Geometry: see drawing. Coordinates: mm, zero at the bounding-box minimum. A direction names the side the tool comes from. Give positions to 0.01 mm unless a question says otherwise; leave off trailing zeros. Order: outer loops, then holes, each group sorted by start corner. A loop starts at its lowest first (then second) coordinate and runs counter-clockwise, first axis right, second up. Notation, with made-up numbers: M 36,-5.5 L 48,-5.5 A21 ccw 48,15.5 Z; hole C 85,36.25 d3. An arc over 180 degrees is marked long. Use a Markdown table: item, result.
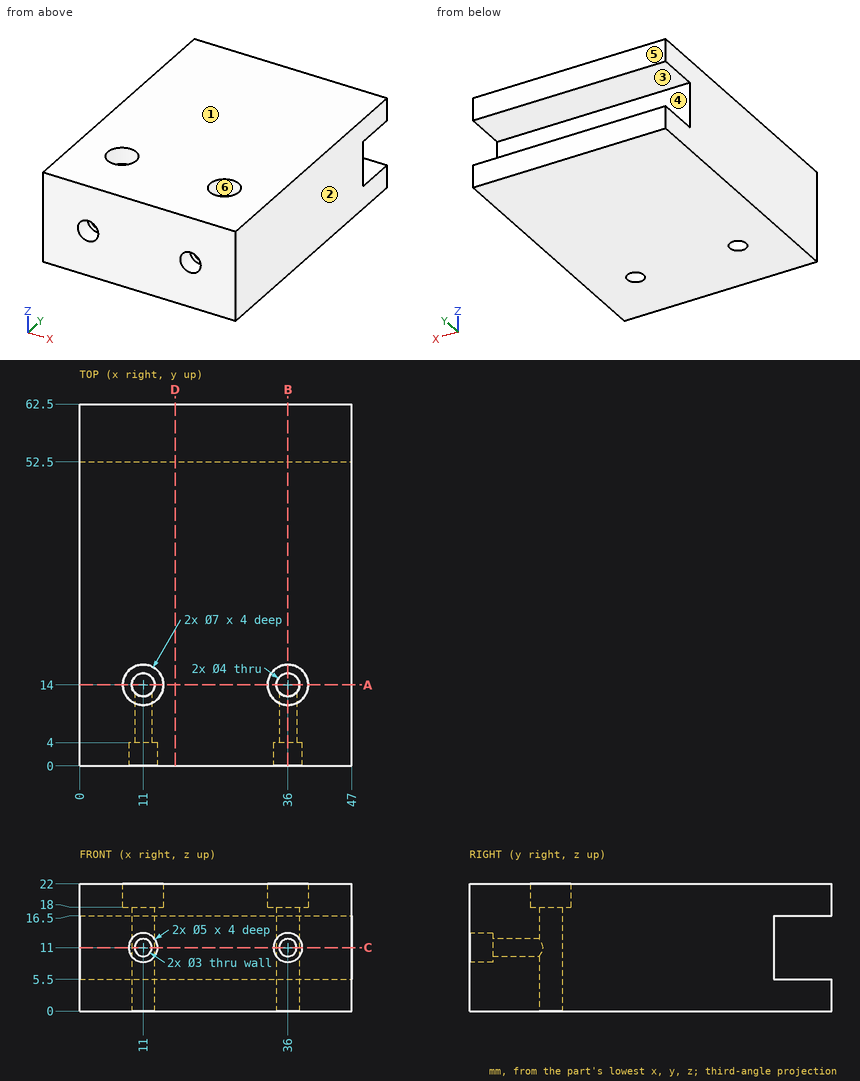
1) Cut plane D-D on x = 16.5. Return loops of the section in (y, z).
Response values:
| item | result |
|---|---|
| outline | M 0,0 L 62.5,0 L 62.5,5.5 L 52.5,5.5 L 52.5,16.5 L 62.5,16.5 L 62.5,22 L 0,22 Z |
2) Material intervals for line 1 (X direction, y = 14, z = 20.5); line 2 (X direction, y = 14, z = 11.5); line 3 (Z direction, x = 11, y = 7.5), sorted ascending. Write a range as from..to.
Response values:
| item | result |
|---|---|
| line 1 | x = 0..7.5, 14.5..32.5, 39.5..47 |
| line 2 | x = 0..9, 13..34, 38..47 |
| line 3 | z = 0..9.5, 12.5..22 |
3) Reachability of the marked faces 5 and 6 from +Z, -Z, +X, -X, +Y, -Y: full face, straight path, thin tool, end or side. Return the list, or none.
Response values:
| item | result |
|---|---|
| face 5 | +Z, -Z, +X, -X, +Y |
| face 6 | +Z |
4) Cut plane B-B on x = 36. Return loops of the section in (y, z).
Response values:
| item | result |
|---|---|
| outline | M 0,0 L 12,0 L 12,9.5 L 4,9.5 L 4,8.5 L 0,8.5 Z; M 0,13.5 L 4,13.5 L 4,12.5 L 12,12.5 L 12,18 L 10.5,18 L 10.5,22 L 0,22 Z; M 16,0 L 62.5,0 L 62.5,5.5 L 52.5,5.5 L 52.5,16.5 L 62.5,16.5 L 62.5,22 L 17.5,22 L 17.5,18 L 16,18 Z |
5) Mould query, pull axis Z, two halves, no side actions, for the marked faces 1, 2, 3 and 4. Classes: released by +Z, released by -Z, zero draft, split by the parting line, or undercut.
Response values:
| item | result |
|---|---|
| face 1 | released by +Z |
| face 2 | zero draft |
| face 3 | undercut |
| face 4 | undercut |
6) Cut plane A-A on y = 14. Return loops of the section in (x, z).
Response values:
| item | result |
|---|---|
| outline | M 0,0 L 9,0 L 9,18 L 7.5,18 L 7.5,22 L 0,22 Z; M 13,0 L 34,0 L 34,18 L 32.5,18 L 32.5,22 L 14.5,22 L 14.5,18 L 13,18 Z; M 38,0 L 47,0 L 47,22 L 39.5,22 L 39.5,18 L 38,18 Z |
7) Cut plane C-C on z = 11. Return loops of the section in (x, y).
Response values:
| item | result |
|---|---|
| outline | M 0,0 L 8.5,0 L 8.5,4 L 9.5,4 L 9.5,12.68 A2 cw long 12.5,12.68 L 12.5,4 L 13.5,4 L 13.5,0 L 33.5,0 L 33.5,4 L 34.5,4 L 34.5,12.68 A2 cw long 37.5,12.68 L 37.5,4 L 38.5,4 L 38.5,0 L 47,0 L 47,52.5 L 0,52.5 Z |
8) First-contact query: pin 1 Ø5 at (x, z) = (36, 11) entering from +Y; pin 2 Ø1.5 at (x, z) = (35.5, 10.5) entering from -Y; pin 3 Ø1.5 at (x, z) = (10, 10) entering from -Y. Flat tips, straight axial feed; report the tip coordinate or a pass-through.
Response values:
| item | result |
|---|---|
| pin 1 | stops at y = 52.5 |
| pin 2 | stops at y = 15.56 |
| pin 3 | stops at y = 4 |
